Can you work these out from the drawing? Everything is in mm from the part's minimum corner. A direction names the side the tool comes from. Round coordinates to 2 decimals unless told otherwise and drop trailing zeros. Write each loop counter-clockwise with the first axis right and the second up, starting at its lowest first coordinate (ties: lowest second). Pieces come first, ordered by that corner, then holes. Notation, with made-up numbers: (57, 85) -> (109, 85) arc R34 cw to (109, 120) -> close; hole circle Ø7 at (81, 82.25). An arc over 180 degrees is marked (long way). Answer as CSV lines item,"result".
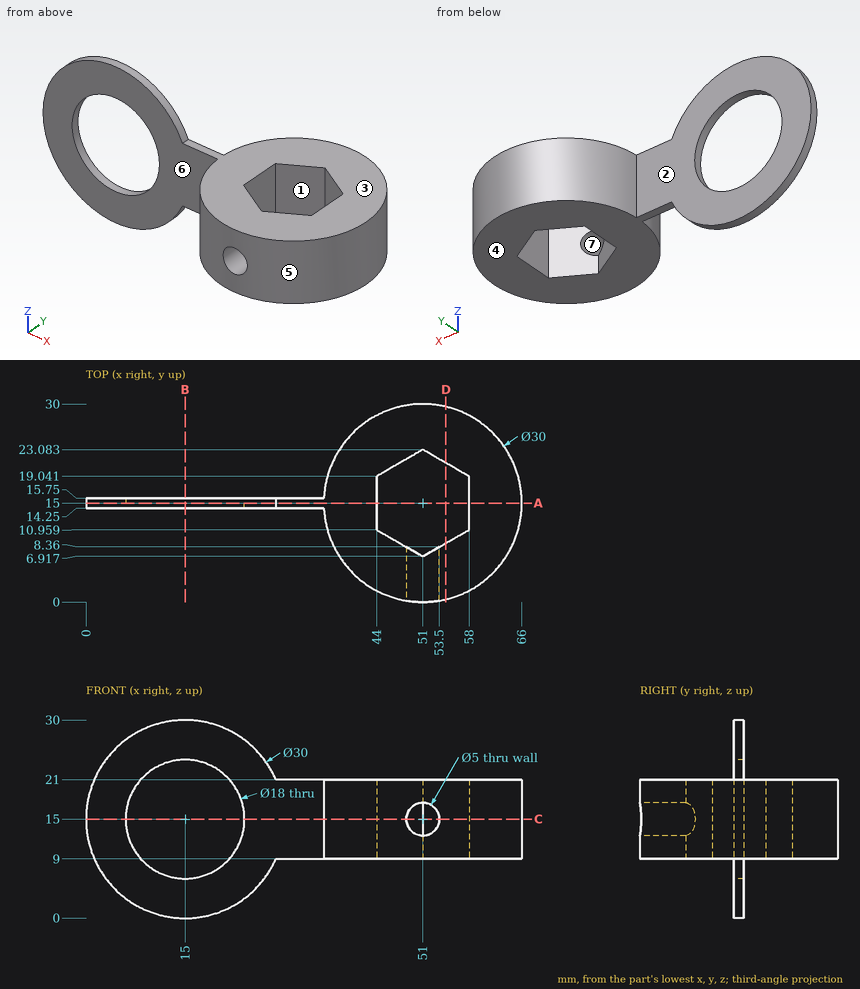
Item 1: If we mould it in two halves opening along X, with no side actions, what happens to the marked faces 5, 6 and 7? For each: pulls with the +X half, pulls with the -X half, needs draft (parallel to the pull), parting line crosses it, or undercut.
Results found:
face 5,"parting line crosses it"
face 6,"needs draft"
face 7,"undercut"
Item 2: Suppose I cut it at C-C, the plane z = 15. List the corners of the cut face in (x, y) for me.
Results found:
outline,"(0, 14.25) -> (6, 14.25) -> (6, 15.75) -> (0, 15.75) -> close; (24, 14.25) -> (36.02, 14.25) arc R15 ccw to (48.5, 0.21) -> (48.5, 8.36) -> (44, 10.96) -> (44, 19.04) -> (51, 23.08) -> (58, 19.04) -> (58, 10.96) -> (53.5, 8.36) -> (53.5, 0.21) arc R15 ccw (long way) to (36.02, 15.75) -> (24, 15.75) -> close"
Item 3: Suppose I cut it at D-D, the plane x = 54.5. List the corners of the cut face in (y, z) for me (1 decimal).
Results found:
outline,"(0.4, 9) -> (8.9, 9) -> (8.9, 21) -> (0.4, 21) -> close; (21.1, 9) -> (29.6, 9) -> (29.6, 21) -> (21.1, 21) -> close"
Item 4: Will these pins go through, and if not, where does the flat tip stop? pin 1 (12 mm diameter, centred on x = 17, y = 26.5, fed in from -Z); pin 2 (5 mm diameter, centred on y = 12, z = 22.5, fed in from +X); pin 3 (6 mm diameter, centred on y = 13.5, z = 4.5, fed in from -X) (1 decimal); pin 4 (5 mm diameter, centred on x = 36, y = 14, fed in from +Z).
Results found:
pin 1,"passes through"
pin 2,"stops at x = 65.97"
pin 3,"stops at x = 2.1"
pin 4,"stops at z = 21"
Item 5: Suppose I cut it at A-A, the plane y = 15. List the corners of the cut face in (x, z) for me.
Results found:
outline,"(28.75, 9) -> (44, 9) -> (44, 21) -> (28.75, 21) arc R15 ccw (long way) to start; (58, 9) -> (66, 9) -> (66, 21) -> (58, 21) -> close; hole circle Ø18 at (15, 15)"
Item 6: For the marked faces 1, 2, 3 and 4, which set-ups out of +Z, -Z, +X, -X, +Y, -Y let a thin tool reach every point of the face, with its end or its side?
Results found:
face 1,"+Z, -Z"
face 2,"+Z, -Z, -X, +Y"
face 3,"+Z, +X, +Y, -Y"
face 4,"-Z, +X, +Y, -Y"
Item 7: I need wall thicknesses on L1, parallel to Z at x = 51, y = 2.5; L2, parallel to Z at x = 15, y = 14.9; L3, parallel to Z at x = 58, y = 26. Which ranges of each line are inside material? Lowest first, please.
Results found:
L1,"z = 9 to 12.5, 17.5 to 21"
L2,"z = 0 to 6, 24 to 30"
L3,"z = 9 to 21"
Item 8: Suppose I cut it at B-B, the plane x = 15. List the corners of the cut face in (y, z) for me.
Results found:
outline,"(14.25, 0) -> (15.75, 0) -> (15.75, 6) -> (14.25, 6) -> close; (14.25, 24) -> (15.75, 24) -> (15.75, 30) -> (14.25, 30) -> close"
